For this review, use the dimensioned drawing (mm, ordinates from the lowest corner) and the shaded views. Round coordinates to 2 decimals unless told otherwise and drop trailing zeros. Order: outer loops, then holes, each group sorted by start corner. A loop starts at its lowest first (then second) coordinate and runs counter-clockwise, first axis right, second up. Notation, with made-up numbers: M 55,44.25 L 72,44.25 A23 ccw 72,58.25 Z; hole C 79.5,53.5 d4. An arc over 180 degrees is marked long. Use a Markdown table: item, result. Add a question column.
1. Consider section A-A on y = 125. State the section outline as (x, z) points.
2. Consider section D-D on z = 1.9. Count the separate pieces of the cut face and the enclosed holes in it, then the cut area to 3 significant figures.
3. Consider section B-B on y = 57. State the section outline as (x, z) points.
4. Consider section C-C on x = 94.5. State the section outline as (y, z) points.
5. To check wall thickness, follow probe 1 along Y at (x, z) = (121, 5.55); probe 2 along X at (y, z) = (111.5, 5.4); probe 3 along Y at (x, z) = (160.5, 2.75). State the ranges of each line that lie inside material, in increasing order.
6. Insertion check: P1, Ø2, axis at x = 148, z = 1.5, coming from the +Y side; P2, Ø3, axis at x = 4, z = 4, coming from the -Y side; P3, Ø3, axis at y = 164, z = 3.5, coming from the +X side. Each pin has a flat end and moves straight along its axis. Give the tip position at first contact, or say it passes through.
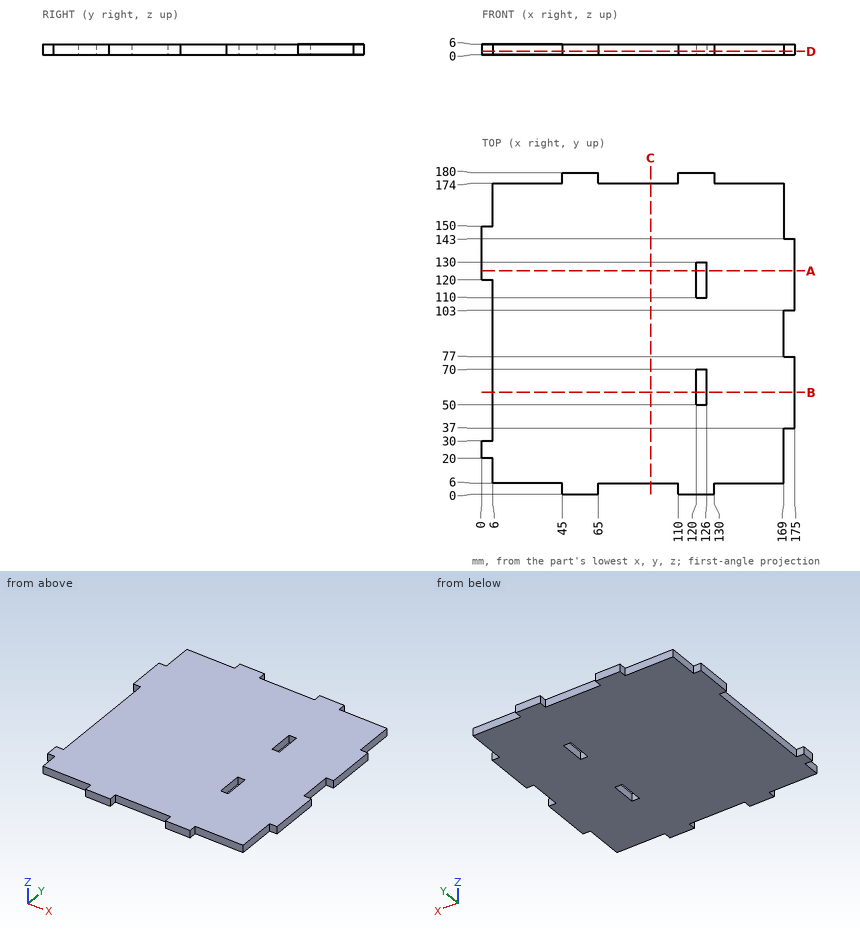
Answer block:
| question | item | result |
|---|---|---|
| 1 | outline | M 0,0 L 120,0 L 120,6 L 0,6 Z; M 126,0 L 175,0 L 175,6 L 126,6 Z |
| 2 | separate pieces | 1 |
| 2 | enclosed holes | 2 |
| 2 | area | 28,300 mm^2 |
| 3 | outline | M 6,0 L 120,0 L 120,6 L 6,6 Z; M 126,0 L 175,0 L 175,6 L 126,6 Z |
| 4 | outline | M 6,0 L 174,0 L 174,6 L 6,6 Z |
| 5 | probe 1 | 0 to 50, 70 to 110, 130 to 180 |
| 5 | probe 2 | 6 to 120, 126 to 175 |
| 5 | probe 3 | 6 to 174 |
| 6 | P1 | y = 174 |
| 6 | P2 | y = 20 |
| 6 | P3 | x = 169 |
